For this review, take the finished solid that the model builds, in its own axes (mm). Face numbers are marked on the shaded views. A direction names the side the tool comes from. Round coordinates to 2 decimals unless told otherwise and drop trailing zeros. Order: outer loops, then holes, each group sorted by start corner. A loop starts at its lowest first (then second) coordinate and runs counter-clockwise, first axis right, second up. Notation, with made-up numbers: M 57.5,4.25 L 69.5,4.25 A21 cw 69.5,15.25 Z; hole C 24.5,52.5 d2. An arc over 180 degrees is marked long. Answer as a JSON object with one key per item and string values.
from build123d import *

# Parameters (mm, degrees)
SKETCH_14_W         = 110
SKETCH_14_H         = 200
EXTRUDE_11_DEPTH    = 15
SKETCH_15_W         = 5
SKETCH_15_H         = 200
EXTRUDE_12_DEPTH    = 30
EXTRUDE_14_DEPTH    = 10
EXTRUDE_15_DEPTH    = 7
SKETCH_19_W         = 4
SKETCH_19_H         = 184
CUT_EXTRUDE_1_DEPTH = 190.489445616
SKETCH_22_W         = 50
SKETCH_22_H         = 2
EXTRUDE_17_DEPTH    = 3
SKETCH_23_W         = 50
SKETCH_23_H         = 2
EXTRUDE_18_DEPTH    = 3
SKETCH_24_W         = 106
SKETCH_24_H         = 9.6
CUT_EXTRUDE_2_DEPTH = 195


with BuildPart() as part:
    # Sketch 14 → Extrude 11 (new body)
    with BuildSketch(Plane.XY):
        with Locations((2.694256757, -17.5)):
            Rectangle(SKETCH_14_W, SKETCH_14_H)
    extrude(amount=EXTRUDE_11_DEPTH)

    # Sketch 15 → Extrude 12 (add)
    with BuildSketch(Plane.XY.offset(15)):
        with Locations((-49.805743243, -17.5)):
            Rectangle(SKETCH_15_W, SKETCH_15_H)
        with Locations((55.194256757, -17.5)):
            Rectangle(SKETCH_15_W, SKETCH_15_H)
    extrude(amount=EXTRUDE_12_DEPTH)

    # Sketch 18 → Extrude 15 (add)
    with BuildSketch(Plane(origin=(0, 82.5, 0), x_dir=(1, 0, 0), z_dir=(0, 1, 0))):
        with BuildLine():
            Line((-52.305743243, -15), (-52.305743243, -45))
            ThreePointArc((-52.305743243, -45), (2.694256757, -100), (57.694256757, -45))
            Line((57.694256757, -45), (57.694256757, -15))
            Line((57.694256757, -15), (-52.305743243, -15))
        make_face()
    extrude(amount=-EXTRUDE_15_DEPTH)

    # Sketch 19 → Cut-Extrude 1 (cut, through all)
    with BuildSketch(Plane.ZY.offset(52.305743243)):
        with Locations((2, -17.5)):
            Rectangle(SKETCH_19_W, SKETCH_19_H)
    extrude(amount=-CUT_EXTRUDE_1_DEPTH, mode=Mode.SUBTRACT)


with BuildPart() as body_2:
    # Sketch 17 → Extrude 14 (new body)
    with BuildSketch(Plane.XZ.offset(117.5)):
        with BuildLine():
            Line((-52.305743243, 15), (-52.305743243, 45))
            ThreePointArc((-52.305743243, 45), (2.694256757, 100), (57.694256757, 45))
            Line((57.694256757, 45), (57.694256757, 15))
            Line((57.694256757, 15), (-52.305743243, 15))
        make_face()
    extrude(amount=-EXTRUDE_14_DEPTH)


    add(part.part)  # Extrude 17 merges part
    # Sketch 22 → Extrude 17 (add)
    with BuildSketch(Plane(origin=(0, -107.5, 0), x_dir=(1, 0, 0), z_dir=(0, 1, 0))):
        with Locations((7.194256757, -76.338233374)):
            Rectangle(SKETCH_22_W, SKETCH_22_H)
    extrude(amount=EXTRUDE_17_DEPTH)

    # Sketch 23 → Extrude 18 (add)
    with BuildSketch(Plane.XZ.offset(-75.5)):
        with Locations((4.598650287, 76.338233374)):
            Rectangle(SKETCH_23_W, SKETCH_23_H)
    extrude(amount=EXTRUDE_18_DEPTH)

    # Sketch 24 → Cut-Extrude 2 (cut)
    with BuildSketch(Plane(origin=(0, 82.5, 0), x_dir=(1, 0, 0), z_dir=(0, 1, 0))):
        with Locations((2.694256757, -10.8)):
            Rectangle(SKETCH_24_W, SKETCH_24_H)
    extrude(amount=-CUT_EXTRUDE_2_DEPTH, mode=Mode.SUBTRACT)


solid = body_2.part
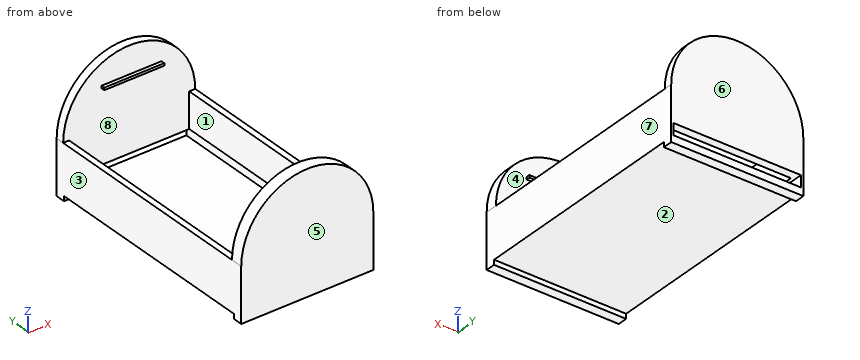
1) Machinability: for the marked faces 1, 2, 3, 4 and 5, which of the approach directions +Z, -Z, +X, -X, +Y, -Y give a long, thin tool a straight path to every point of the face, cutting with its end or side? Answer none if there is none.
Geometry check:
{"face 1": "+Z", "face 2": "-Z, +X, -X", "face 3": "+Z, -Z, -X, +Y, -Y", "face 4": "none", "face 5": "+Z, -Z, +X, -X, -Y"}
2) Insertion check: P1, Ø2.5, axis at x = 54.5, y = -23.5, coming from the +Z side; P2, Ø2, axis at y = 73.5, z = 76.5, coming from the -X side; P3, Ø1, axis at y = -106.5, z = 76.5, coming from the -X side. Each pin has a flat end and moves straight along its axis. Give the tip position at first contact, or say it passes through.
Geometry check:
{"P1": "stops at z = 45", "P2": "stops at x = -20.4", "P3": "stops at x = -17.81"}
3) For L1, parallel to X at y = -2.5, z = 38.5; L2, parallel to Y at x = 32.5, z = 33; L3, parallel to X at y = -0.5, z = 9, list the stretches that pass through material, from the lowest coordinate up.
Geometry check:
{"L1": "x = -52.31 to -47.31, 52.69 to 57.69", "L2": "y = -117.5 to -107.5, 75.5 to 82.5", "L3": "x = -52.31 to -50.31, 55.69 to 57.69"}
4) Add section D-D on z = 12.5. State the section outline as (x, y) points, and give its area (3 significant figures).
Geometry check:
{"outline": "M -52.31,-117.5 L 57.69,-117.5 L 57.69,82.5 L 55.69,82.5 L 55.69,-112.5 L -50.31,-112.5 L -50.31,82.5 L -52.31,82.5 Z", "area": "1,330 mm²"}
5) Mouldability with a two-part tool opening along X and no side actions: class the marked faces 6, 7 and 8 as +X half, -X half, draft (parallel to the pull), parting line (faces both ways), or undercut.
Geometry check:
{"face 6": "draft", "face 7": "+X half", "face 8": "undercut"}
6) Add section B-B on x = -8. State the section outline as (y, z) points, and give its area (3 significant figures).
Geometry check:
{"outline": "M -117.5,0 L -109.5,0 L -109.5,4 L 74.5,4 L 74.5,0 L 82.5,0 L 82.5,6 L -112.5,6 L -112.5,15.6 L -107.5,15.6 L -107.5,75.34 L -104.5,75.34 L -104.5,77.34 L -107.5,77.34 L -107.5,98.95 L -117.5,98.95 Z; M 72.5,75.34 L 75.5,75.34 L 75.5,15.6 L 82.5,15.6 L 82.5,98.95 L 75.5,98.95 L 75.5,77.34 L 72.5,77.34 Z", "area": "1,940 mm²"}
7) Add section C-C on z = 89. State the section outline as (x, y) points.
Geometry check:
{"outline": "M -30.31,-117.5 L 35.69,-117.5 L 35.69,-107.5 L -30.31,-107.5 Z; M -30.31,75.5 L 35.69,75.5 L 35.69,82.5 L -30.31,82.5 Z"}
8) Add section A-A on y = -14.5. State the section outline as (x, z) points, and give its area (3 significant figures).
Geometry check:
{"outline": "M -52.31,4 L 57.69,4 L 57.69,45 L 52.69,45 L 52.69,15.6 L 55.69,15.6 L 55.69,6 L -50.31,6 L -50.31,15.6 L -47.31,15.6 L -47.31,45 L -52.31,45 Z", "area": "552 mm²"}
